Check sheet for the drawn part. Datum: minimum x, y, z corner. Units: mm. A direction names the side the tool comes from. Round coordinates to 2 decimals unless told otherwise and drop trailing zeros. Order: outer loops, then holes, each group sorted by start corner. A loop starts at its lowest first (then second) coordinate and runs counter-clockwise, first axis right, second up.
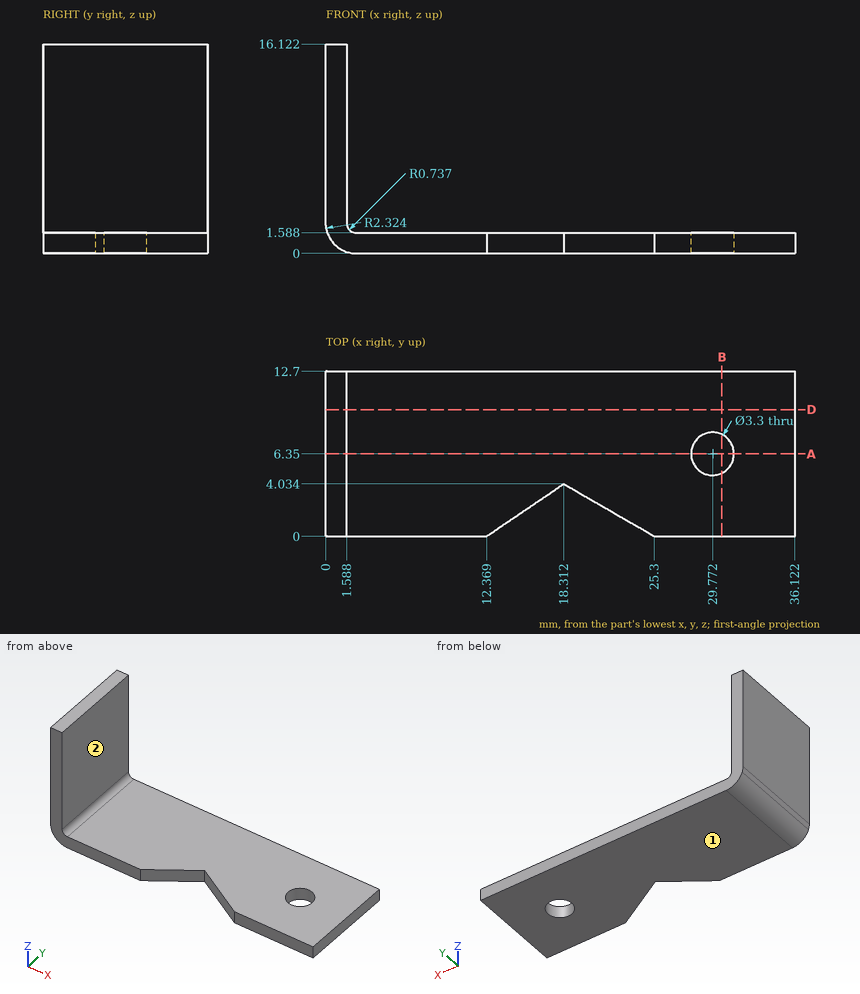
(1) Material ranges on line 1 (Z direction, x = 10, y = 10.5), recorded low to high.
Returned:
line 1: z = 0 to 1.59
(2) Sectioned sample at B-B, the plane x = 30.5. Record the cut outline in (y, z).
Returned:
outline: (0, 0) - (4.87, 0) - (4.87, 1.59) - (0, 1.59) - close; (7.83, 0) - (12.7, 0) - (12.7, 1.59) - (7.83, 1.59) - close
(3) Set-up check for the marked faces 1 and 2: record each of +Z, -Z, +X, -X, +Y, -Y from which the full face is reachable in a straight line by a thin tool's end or side.
Returned:
face 1: -Z, +X, -X, +Y, -Y
face 2: +Z, +X, +Y, -Y
(4) Depth check by flat-ended pin: P1, Ø4, axis at y = 8, z = 7, coming from the +X side; P2, Ø6, axis at x = 26, y = 7, coming from the +Z side. Enter the tip coordinate at first touch or a pass-through.
Returned:
P1: stops at x = 1.59
P2: stops at z = 1.59
(5) Sectioned sample at D-D, the plane y = 9.75. Record the cut outline in (x, z) (1 decimal).
Returned:
outline: (0, 2.3) arc R2.3 ccw to (2.3, 0) - (36.1, 0) - (36.1, 1.6) - (2.3, 1.6) arc R0.7 cw to (1.6, 2.3) - (1.6, 16.1) - (0, 16.1) - close
(6) Sectioned sample at A-A, the plane y = 6.35. Record the cut outline in (x, z) (1 decimal).
Returned:
outline: (0, 2.3) arc R2.3 ccw to (2.3, 0) - (28.1, 0) - (28.1, 1.6) - (2.3, 1.6) arc R0.7 cw to (1.6, 2.3) - (1.6, 16.1) - (0, 16.1) - close; (31.4, 0) - (36.1, 0) - (36.1, 1.6) - (31.4, 1.6) - close
